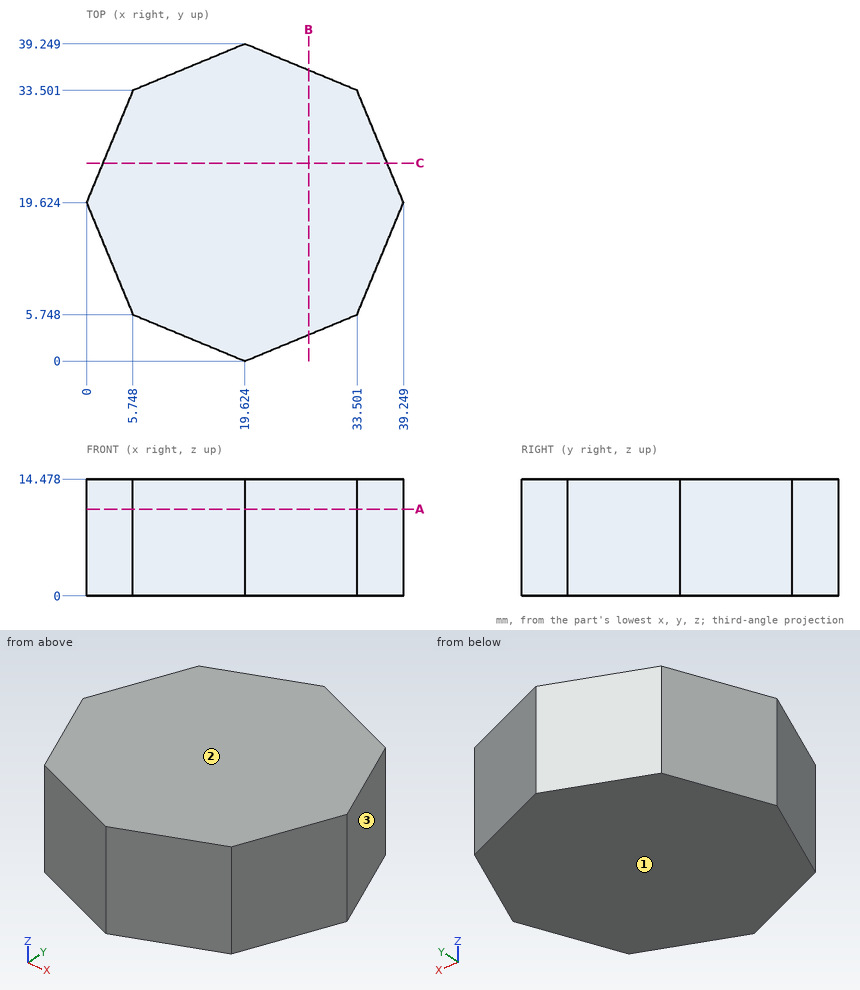
Can you work these out from the drawing? Everything is in mm from the part's minimum corner. Coordinates: 2 decimals unless noted, no trailing zeros. Loops run counter-clockwise (first coordinate to the right, second up) from the corner with the lowest first, then second, coordinate; pieces in that order, holes last.
1. Imagine slicing it at C-C, the plane y = 24.5. Please give me the cut outline in (x, z).
2. For P1, Ø6, axis at y = 16.5, z = 12.5, coming from the -X side; P2, Ø4, axis at x = 11.5, z = 12, coming from the +Y side; P3, Ø1, axis at x = 4.5, y = 33.5, coming from the +Z side, each with a flat end and sliding along its axis, tell me the tip position at first contact or that it passes through.
3. If we mould it in two halves opening along Z, with no side actions, what happens to the marked faces 1, 2 and 3? For each: pulls with the +Z half, pulls with the -Z half, needs draft (parallel to the pull), parting line crosses it, or undercut.
4. I need wall thicknesses on L1, parallel to Y at x = 22, z = 11.5 (1 decimal); L2, parallel to X at y = 4.5, z = 9 (1 decimal); L3, parallel to Y at x = 22.5, z = 9.5. Which ranges of each line are inside material? Lowest first, please.
5. Imagine slicing it at A-A, the plane z = 10.75. Please give me the cut outline in (x, y) (1 decimal).
6. Imagine slicing it at B-B, the plane x = 27.5. Please give me the cut outline in (y, z), and give its area (3 significant figures).
Taken from the geometry:
1. outline: (2.02, 0) - (37.23, 0) - (37.23, 14.48) - (2.02, 14.48) - close
2. P1: stops at x = 0.05
2. P2: stops at y = 36.71
2. P3: passes through
3. face 1: pulls with the -Z half
3. face 2: pulls with the +Z half
3. face 3: needs draft
4. L1: y = 1 to 38.3
4. L2: x = 8.8 to 30.5
4. L3: y = 1.19 to 38.06
5. outline: (0, 19.6) - (5.7, 5.7) - (19.6, 0) - (33.5, 5.7) - (39.2, 19.6) - (33.5, 33.5) - (19.6, 39.2) - (5.7, 33.5) - close
6. outline: (3.26, 0) - (35.99, 0) - (35.99, 14.48) - (3.26, 14.48) - close
6. area: 474 mm2
